Source: CAD feature listing. Evaluate the final solid. Frame: model axes, mm. Round coordinates to 2 decimals unless told otherwise and drop trailing zeros. Loops run counter-clockwise (first coordinate to the right, second up) from the corner with the lowest first, then second, coordinate; pieces in that order, holes last. Notation, with made-up numbers: M -18.75,87 L -4.75,87 A17 ccw -4.75,111 Z; hole C 47,69 d5. An arc over 180 degrees is marked long. Answer as a JSON object with one key per item and string values.
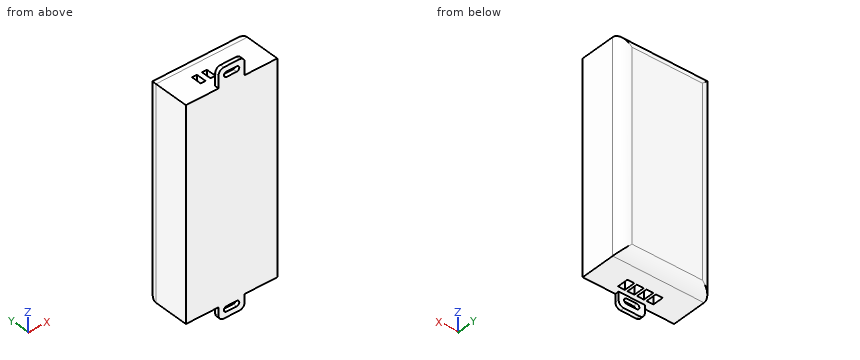
from build123d import *

# Parameters (mm, degrees)
SKETCH1_W           = 44.45
SKETCH1_H           = 101.6
BOSS_EXTRUDE1_DEPTH = 22.225
FILLET1_R           = 5.08
SKETCH2_R           = 2.981516586
CUT_EXTRUDE1_DEPTH  = 12.7
SKETCH3_W           = 2.38773998
SKETCH3_H           = 4.914706725
SKETCH3_W_2         = 2.387739981
CUT_EXTRUDE2_DEPTH  = 7.62
SKETCH4_W           = 3.327455713
SKETCH4_H           = 5.359264955
SKETCH4_W_2         = 3.327455714
CUT_EXTRUDE3_DEPTH  = 7.62
BOSS_EXTRUDE2_DEPTH = 1.905


with BuildPart() as part:
    # Sketch1 → Boss-Extrude1 (new body)
    with BuildSketch(Plane(origin=(0, 0, 0), x_dir=(1, 0, 0), z_dir=(0, 1, 0))):
        with Locations((22.225, 50.8)):
            Rectangle(SKETCH1_W, SKETCH1_H)
    extrude(amount=BOSS_EXTRUDE1_DEPTH)

    # Fillet1
    fillet1_edges = [part.edges().sort_by_distance(p)[0] for p in [
        (44.45, 22.225, -50.8),
        (22.225, 22.225, -101.6),
        (0, 22.225, -50.8),
        (22.225, 22.225, 0),
    ]]
    fillet(fillet1_edges, radius=FILLET1_R)

    # Sketch2 → Cut-Extrude1 (cut)
    with BuildSketch(Plane.XY):
        with Locations((27.915098323, 6.294196756)):
            Circle(SKETCH2_R)
    extrude(amount=-CUT_EXTRUDE1_DEPTH, mode=Mode.SUBTRACT)

    # Sketch3 → Cut-Extrude2 (cut)
    with BuildSketch(Plane.XY):
        with Locations((14.031826574, 9.129741005)):
            Rectangle(SKETCH3_W, SKETCH3_H)
        with Locations((18.859604577, 9.129741005)):
            Rectangle(SKETCH3_W_2, SKETCH3_H)
    extrude(amount=-CUT_EXTRUDE2_DEPTH, mode=Mode.SUBTRACT)

    # Sketch4 → Cut-Extrude3 (cut)
    with BuildSketch(Plane(origin=(0, 0, -101.6), x_dir=(-1, 0, 0), z_dir=(0, 0, -1))):
        with Locations((-29.15965328, 6.872202453)):
            Rectangle(SKETCH4_W, SKETCH4_H)
        with Locations((-24.536551093, 6.872202453)):
            Rectangle(SKETCH4_W_2, SKETCH4_H)
        with Locations((-19.913448907, 6.872202453)):
            Rectangle(SKETCH4_W_2, SKETCH4_H)
        with Locations((-15.290346721, 6.872202453)):
            Rectangle(SKETCH4_W, SKETCH4_H)
    extrude(amount=-CUT_EXTRUDE3_DEPTH, mode=Mode.SUBTRACT)

    # Sketch5 → Boss-Extrude2 (add)
    with BuildSketch(Plane.XZ):
        with BuildLine():
            Line((15.875, 0), (15.875, 6.058263516))
            ThreePointArc((15.875, 6.058263516), (16.618948776, 7.85431474), (18.415, 8.598263516))
            Line((18.415, 8.598263516), (26.035, 8.598263516))
            ThreePointArc((26.035, 8.598263516), (27.831051224, 7.85431474), (28.575, 6.058263516))
            Line((28.575, 6.058263516), (28.575, 0))
            Line((28.575, 0), (15.875, 0))
        make_face()
        with BuildLine():
            Line((19.751425895, 5.984747985), (24.698574105, 5.984747985))
            ThreePointArc((24.698574105, 5.984747985), (25.952772297, 4.730549793), (24.698574105, 3.476351601))
            Line((24.698574105, 3.476351601), (19.751425895, 3.476351601))
            ThreePointArc((19.751425895, 3.476351601), (18.497227703, 4.730549793), (19.751425895, 5.984747985))
        make_face(mode=Mode.SUBTRACT)
    boss_extrude2 = extrude(amount=-BOSS_EXTRUDE2_DEPTH)

    # Mirror2: Boss-Extrude2 across plane
    add(boss_extrude2.mirror(Plane.XY.offset(-49.738094236)))


solid = part.part
Item 1: Section D-D on x = 41.5. Return the cut outline in (y, z) (3 decimals).
Answer sheet:
{"outline": "M 0,-101.6 L 17.145,-101.6 A5.08 ccw 21.757,-98.65 L 21.757,-2.95 A5.08 ccw 17.145,0 L 0,0 Z"}
Item 2: Section B-B on x = 11. Return the cut outline in (y, z) (3 decimals).
Answer sheet:
{"outline": "M 0,-101.6 L 17.145,-101.6 A5.08 ccw 22.225,-96.52 L 22.225,-5.08 A5.08 ccw 17.145,0 L 0,0 Z"}
Item 3: Line query: probe 1 along X at (y, z) = (9, -98); probe 2 along Z at (x, y) = (19, 5); probe 3 along Z at (x, y) = (25, 15.75). Output: solid intervals per line, ascending. Write a range as from..to.
Answer sheet:
{"probe 1": "x = 0..13.63, 16.95..18.25, 21.58..22.87, 26.2..27.5, 30.82..44.45", "probe 2": "z = -93.98..0", "probe 3": "z = -101.6..0"}
Item 4: Contact query for flat-ended pins moving along their axis: pin 1 Ø2 at (y, z) = (1, 4.5) entering from +X (3 decimals); pin 2 Ø6 at (x, y) = (20.5, 3.5) entering from +Z; pin 3 Ø2.5 at (x, z) = (20.5, -99.5) entering from +Y; pin 4 Ø1.5 at (x, y) = (7.5, 15) entering from -Z. Output: stop coordinate, or through.
Answer sheet:
{"pin 1": "stops at x = 28.575", "pin 2": "stops at z = 8.6", "pin 3": "stops at y = 21.92", "pin 4": "stops at z = -101.6"}
Item 5: Section A-A on z = -100. Return the cut outline in (x, y) (3 decimals), then the cut area to 3 significant figures.
Answer sheet:
{"outline": "M 0,0 L 44.45,0 L 44.45,17.145 A5.08 ccw 42.85,20.846 L 1.6,20.846 A5.08 ccw 0,17.145 Z; hole M 13.627,4.193 L 16.954,4.193 L 16.954,9.552 L 13.627,9.552 Z; hole M 18.25,4.193 L 21.577,4.193 L 21.577,9.552 L 18.25,9.552 Z; hole M 22.873,4.193 L 26.2,4.193 L 26.2,9.552 L 22.873,9.552 Z; hole M 27.496,4.193 L 30.823,4.193 L 30.823,9.552 L 27.496,9.552 Z", "area": "852 mm²"}
Item 6: Section C-C on y = 15.5. Return the cut outline in (x, z).
Answer sheet:
{"outline": "M 0,-101.6 L 44.45,-101.6 L 44.45,0 L 0,0 Z"}
